from build123d import *

# Parameters (mm, degrees)
CUT_EXTRUDE1_REACH = 11.5
SKETCH2_R          = 1.5
CHAMFER1_SIZE      = 0.5


with BuildPart() as part:
    # Sketch1 → Revolve1 (revolve)
    with BuildSketch(Plane.XY):
        Polygon((-12.5, 4), (0, 4), (0, 2.5), (12.5, 2.5), (12.5, 9.5), (-12.5, 9.5), align=None)
    revolve(axis=Axis((-12.5, 0, 0), (1, 0, 0)))

    # Sketch2 → Cut-Extrude1 (cut, up to next)
    with BuildSketch(Plane(origin=(0, 0, 0), x_dir=(1, 0, 0), z_dir=(0, 1, 0)), mode=Mode.PRIVATE) as cut_extrude1_sk1:
        with Locations((-9.5, 0)):
            Circle(SKETCH2_R)
    cut_extrude1_tool1 = extrude(cut_extrude1_sk1.sketch, amount=CUT_EXTRUDE1_REACH, mode=Mode.PRIVATE) & part.part
    add(cut_extrude1_tool1.solids().sort_by_distance((-9.5, 0, 0))[0], mode=Mode.SUBTRACT)
    # Sketch2 → Cut-Extrude1 (cut, up to next)
    with BuildSketch(Plane(origin=(0, 0, 0), x_dir=(1, 0, 0), z_dir=(0, 1, 0)), mode=Mode.PRIVATE) as cut_extrude1_sk2:
        with Locations((9.5, 0)):
            Circle(SKETCH2_R)
    cut_extrude1_tool2 = extrude(cut_extrude1_sk2.sketch, amount=CUT_EXTRUDE1_REACH, mode=Mode.PRIVATE) & part.part
    add(cut_extrude1_tool2.solids().sort_by_distance((9.5, 0, 0))[0], mode=Mode.SUBTRACT)

    # Chamfer1
    chamfer1_edges = [part.edges().sort_by_distance(p)[0] for p in [
        (-12.5, -9.5, 0),
        (12.5, -9.5, 0),
    ]]
    chamfer(chamfer1_edges, length=CHAMFER1_SIZE)


solid = part.part
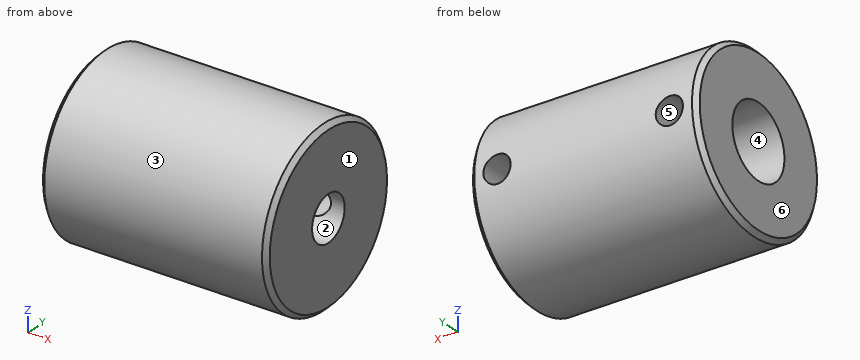
Model file for the job. Use its own axes, mm. Face numbers are marked on the shaded views. A direction names the side the tool comes from. Round coordinates to 2 decimals unless told otherwise and drop trailing zeros. Loops run counter-clockwise (first coordinate to the right, second up) from the corner with the lowest first, then second, coordinate; pieces in that order, holes last. Notation, with made-up numbers: (12, -14) -> (41, -14) arc R22 cw to (41, 22) -> close; hole circle Ø5 at (15.5, 29). An arc over 180 degrees is marked (long way). Answer as CSV lines item,"result". Start each with the question number.
1) Slice it at B-B (z = 0). List the corners of the cut face in (x, y), plus the area to 4 significant figures.
2) Slice it at A-A (y = 0). List the corners of the cut face in (x, z).
3) Mould opens along Z. For the marked faces 1, 2, 3 and 4 say: +Z half, -Z half, draft (parallel to the pull), parting line (faces both ways), or undercut.
4) Slice it at D-D (x = -9.5). List the corners of the cut face in (y, z).
5) Tool access for the marked faces 5 and 6: list every direction of +Z, -Z, +X, -X, +Y, -Y with a clear straight run to the whole face (end or side of a thin tool).
6) Pin check, flat tips, straight feed: P1, Ø2, axis at x = -8.5, y = 2.5, coming from the -Z side; P2, Ø5, axis at x = 9.5, z = 0, coming from the +Y side; P3, Ø6, axis at x = 4.5, z = 6.5, coming from the -Y side; P4, Ø6.5, axis at y = 0, z = 0, coming from the -X side. Stop position of each tip, or through.
7) Slice it at C-C (x = 4.5). List the corners of the cut face in (y, z), plus the area to 3 significant figures.
8) Probe line 1 along Z through (x, y) = (5.5, 0); line 2 along Y through (x, z) = (-5.5, 0.25); line 3 along X through (y, z) = (-1, 2.5). List the from-to ranges inside material, lowest first.
Filled in:
1,outline,"(-12.5, -9) -> (-12, -9.5) -> (12, -9.5) -> (12.5, -9) -> (12.5, -2.5) -> (0, -2.5) -> (0, -4) -> (-12.5, -4) -> close; (-12.5, 4) -> (-11, 4) -> (-11, 9.5) -> (-12, 9.5) -> (-12.5, 9) -> close; (-8, 4) -> (0, 4) -> (0, 2.5) -> (8, 2.5) -> (8, 9.5) -> (-8, 9.5) -> close; (11, 2.5) -> (12.5, 2.5) -> (12.5, 9) -> (12, 9.5) -> (11, 9.5) -> close"
1,area,"274.5 mm2"
2,outline,"(-12.5, -9) -> (-12, -9.5) -> (12, -9.5) -> (12.5, -9) -> (12.5, -2.5) -> (0, -2.5) -> (0, -4) -> (-12.5, -4) -> close; (-12.5, 4) -> (0, 4) -> (0, 2.5) -> (12.5, 2.5) -> (12.5, 9) -> (12, 9.5) -> (-12, 9.5) -> (-12.5, 9) -> close"
3,face 1,"draft"
3,face 2,"undercut"
3,face 3,"parting line"
3,face 4,"undercut"
4,outline,"(3.71, -1.5) arc R4 cw (long way) to (3.71, 1.5) -> (9.38, 1.5) arc R9.5 ccw (long way) to (9.38, -1.5) -> close"
5,face 5,"+Y"
5,face 6,"+Z, -Z, -X, +Y, -Y"
6,P1,"stops at z = -9.38"
6,P2,"stops at y = 9.5"
6,P3,"stops at y = -8.83"
6,P4,"stops at x = 0"
7,outline,"circle Ø19 at (0, 0); hole circle Ø5 at (0, 0)"
7,area,"264 mm2"
8,line 1,"z = -9.5 to -2.5, 2.5 to 9.5"
8,line 2,"y = -9.5 to -3.99, 3.99 to 9.5"
8,line 3,"x = 0 to 12.5"
